The model under review builds one solid part; all positions refer to its coordinate system, in mm. Face numbers are marked on the shaded views. Coordinates: 2 decimals unless noted, no trailing zeros. Order: outer loops, then holes, each group sorted by start corner. A loop starts at its lowest first (then second) coordinate and runs counter-clockwise, first axis right, second up. Notation, with made-up numbers: M 53.25,-24 L 59.25,-24 A20 ccw 59.25,-9 Z; hole C 0.25,15 d3. An arc over 180 degrees is marked long. Answer in a Markdown table with one row per item.
Autodesk Inventor part; units mm, degrees
ref_plane "YZ Plane" through (0, 0, 0) normal (1, 0, 0) x (0, 1, 0)
ref_plane "XZ Plane" through (0, 0, 0) normal (0, 1, 0) x (-1, 0, 0)
ref_plane "XY Plane" through (0, 0, 0) normal (0, 0, 1) x (1, 0, 0)
sketch "Sketch2" plane through (0, 0, 0) normal (0, 0, 1) x (1, 0, 0)
  circle A0 centre (0, 0) radius 6
  line L0 (-11, 0) -> (11, 0)
  line L1 (11, 0) -> (11, -10)
  line L2 (11, -10) -> (-11, -10)
  line L3 (-11, -10) -> (-11, 0)
  circle A1 centre (0, 0) radius 9
  point P0 (6, 0)
  point P1 (-6, 0)
  dimension "d0" = 12
  dimension "d1" = 11
  dimension "d2" = 11
  dimension "d3" = 10
  dimension "d4" = 3
extrude "Extrusion1" add sketch "Sketch2" along normal blind 10 contours L0 A1 A0 | L0 L1 L2 L3 A1 picked at (-7.9128, -0.7179)
sketch "Sketch3" plane through (6, 0, 0) normal (0, 1, 0) x (1, 0, 0)
  circle A0 centre (2, -5) radius 1.6
  line L0 (5, 0) -> (5, -10)
  line L1 (5, 0) -> (0, 0)
  circle A1 centre (-14, -5) radius 1.6
  line L2 (-17, 0) -> (-17, -10)
  line L3 (-12, 0) -> (-17, 0)
  point P0 (-6, 0)
  dimension "d7" = 3.2
  dimension "d8" = 3
  dimension "d9" = 5
  dimension "d10" = 3.2
  dimension "d11" = 3
  dimension "d12" = 5
extrude "Extrusion2" cut sketch "Sketch3" against normal blind 10
sketch "Sketch4" plane through (-11, -10, 0) normal (0, -1, 0) x (1, 0, 0)
  circle A0 centre (11, 5) radius 1.6
  line L0 (0, 0) -> (22, 0)
  point P0 (11, 0)
  dimension "d15" = 3.2
  dimension "d16" = 5
extrude "Extrusion3" cut sketch "Sketch4" against normal blind 10
properties part number "Tube_mount_centering"
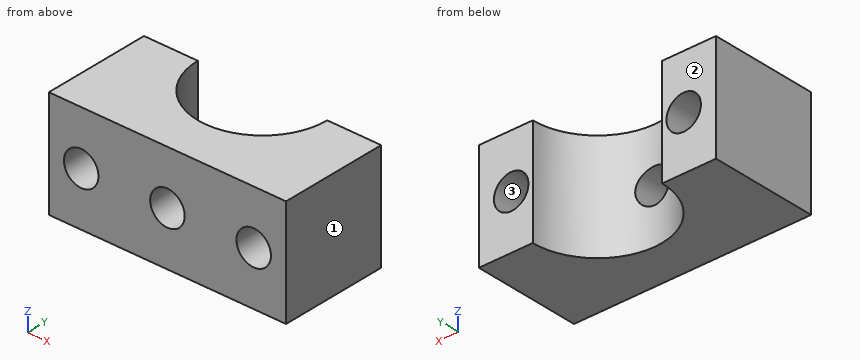
(1) To check wall thickness, follow line 1 (Z direction, x = 8, y = -4.25); line 2 (X direction, y = -7.6, z = 5); line 3 (X direction, y = -7.75, z = 6). State the ranges of each line that lie inside material, in increasing order. Write a range as [from, to].
Report:
| item | result |
|---|---|
| line 1 | [0, 3.4], [6.6, 10] |
| line 2 | [-11, -9.6], [-6.4, -1.6], [1.6, 6.4], [9.6, 11] |
| line 3 | [-11, -9.25], [-6.75, -1.25], [1.25, 6.75], [9.25, 11] |
(2) The part is to be moulded in two halves that separate along X. For the marked faces 1, 2 and 3, say which applies: +X half, -X half, draft (parallel to the pull), parting line (faces both ways), or undercut.
Report:
| item | result |
|---|---|
| face 1 | +X half |
| face 2 | draft |
| face 3 | undercut |
(3) Insertion check: P1, Ø3.5, axis at x = 0, z = 5, coming from the +Y side. The pin has a flat end and moves straight along its axis. Give the tip position at first contact, or say it passes through.
Report:
| item | result |
|---|---|
| P1 | y = -5.74 |
(4) Take a section at A-A (x = 0). Write out the cut boundary in (y, z), then the cut area to 3 significant figures.
Report:
| item | result |
|---|---|
| outline | M -10,0 L -6,0 L -6,3.4 L -10,3.4 Z; M -10,6.6 L -6,6.6 L -6,10 L -10,10 Z |
| area | 27.2 mm^2 |
(5) Take a section at B-B (y = -2.75). Write out the cut boundary in (x, z), then the cut area to 3 significant figures.
Report:
| item | result |
|---|---|
| outline | M -11,0 L -5.33,0 L -5.33,10 L -11,10 Z; M 5.33,0 L 11,0 L 11,10 L 5.33,10 Z; hole C -8,5 d3.2; hole C 8,5 d3.2 |
| area | 97.3 mm^2 |
(6) Take a section at D-D (z = 1.75). Write out the cut boundary in (x, y), then the cut area to 3 significant figures.
Report:
| item | result |
|---|---|
| outline | M -11,-10 L 11,-10 L 11,0 L 6,0 A6 cw -6,0 L -11,0 Z |
| area | 163 mm^2 |
(7) Take a section at C-C (z = 6). Write out the cut boundary in (x, y).
Report:
| item | result |
|---|---|
| outline | M -11,-10 L -9.25,-10 L -9.25,0 L -11,0 Z; M -6.75,-10 L -1.25,-10 L -1.25,-5.87 A6 cw -6,0 L -6.75,0 Z; M 1.25,-10 L 6.75,-10 L 6.75,0 L 6,0 A6 cw 1.25,-5.87 Z; M 9.25,-10 L 11,-10 L 11,0 L 9.25,0 Z |
